The listing builds one solid part. Answer for the finished solid, in the listing's coordinates (mm). A direction names the side the tool comes from. Give positions to 0.01 mm unless a question says otherwise; leave off trailing zeros. Write each loop counter-clockwise with the first axis right and the second up, starting at its lowest first coordinate (ties: lowest second). Pieces come first, ordered by that corner, then holes. Notation, with made-up numbers: M 75,74.5 L 100,74.5 A36 cw 100,111.5 Z; hole C 63,46 d1. An arc over 180 degrees is marked long. Return JSON: item names as keys, results as strings.
from build123d import *

# Parameters (mm, degrees)
SKETCH1_R           = 6.35
BOSS_EXTRUDE1_DEPTH = 17.5
CUT_EXTRUDE1_DEPTH  = 12.8
CHAMFER1_SIZE       = 2
SKETCH4_R           = 3.5
BOSS_EXTRUDE2_DEPTH = 25
SKETCH8_R           = 1.625
CUT_EXTRUDE4_DEPTH  = 30
SKETCH7_R           = 2.5
CUT_EXTRUDE3_DEPTH  = 3.5
SKETCH9_R           = 4
SKETCH9_R_2         = 1.625
BOSS_EXTRUDE3_DEPTH = 5
SKETCH11_R          = 2.75
CUT_EXTRUDE5_DEPTH  = 3
SKETCH12_R          = 1.625
CUT_EXTRUDE6_DEPTH  = 101.436547133
BOSS_EXTRUDE4_DEPTH = 3.7
SKETCH14_R          = 6.35
CUT_EXTRUDE7_DEPTH  = 3.7
CUT_EXTRUDE8_REACH  = 100.805
SKETCH15_W          = 2
SKETCH15_H          = 32.561115391
SKETCH15_H_2        = 13.634806385
SKETCH16_W          = 2
SKETCH16_H          = 5.291502622
CUT_EXTRUDE9_DEPTH  = 20
CUT_EXTRUDE10_REACH = 102.437
SKETCH17_R          = 1.5
CUT_EXTRUDE11_REACH = 102.437
SKETCH18_W          = 1.2
SKETCH18_H          = 8


with BuildPart() as part:
    # Sketch1 → Boss-Extrude1 (new, symmetric)
    with BuildSketch(Plane(origin=(0, 0, 0), x_dir=(0, 0, -1), z_dir=(1, 0, 0))):
        with BuildLine():
            Line((-75, -17.5), (75, -17.5))
            ThreePointArc((75, -17.5), (91.201851746, -6.614378278), (87.247448714, 12.5))
            Line((87.247448714, 12.5), (-69.247448714, 12.5))
            Line((-69.247448714, 12.5), (-69.247448714, 17.5))
            Line((-69.247448714, 17.5), (-75, 17.5))
            ThreePointArc((-75, 17.5), (-92.5, 0), (-75, -17.5))
        make_face()
        with Locations((-75, 0)):
            Circle(SKETCH1_R, mode=Mode.SUBTRACT)
        with Locations((75, 0)):
            Circle(SKETCH1_R, mode=Mode.SUBTRACT)
    extrude(amount=BOSS_EXTRUDE1_DEPTH, both=True)

    # Sketch3 → Cut-Extrude1 (cut, symmetric)
    with BuildSketch(Plane(origin=(0, 0, 0), x_dir=(0, 0, -1), z_dir=(1, 0, 0))):
        with BuildLine():
            Line((-55, -12.5), (75, -12.5))
            ThreePointArc((75, -12.5), (86.858541226, -3.952847075), (82.5, 10))
            Line((82.5, 10), (82.5, 17.5))
            Line((82.5, 17.5), (-92.5, 17.5))
            Line((-92.5, 17.5), (-92.5, -17.5))
            Line((-92.5, -17.5), (-55, -17.5))
            Line((-55, -17.5), (-55, -12.5))
        make_face()
    extrude(amount=CUT_EXTRUDE1_DEPTH, both=True, mode=Mode.SUBTRACT)

    # Chamfer1
    chamfer1_edges = [part.edges().sort_by_distance(p)[0] for p in [
        (17.5, -6.614378278, -91.201851746),
        (17.5, 17.5, 72.123724357),
        (0, -12.5, 55),
        (17.5, 0, 92.5),
        (-17.5, 17.5, 72.123724357),
        (-17.5, -6.614378278, -91.201851746),
        (-17.5, -17.5, 0),
        (-17.5, 0, 92.5),
        (17.5, -17.5, 0),
    ]]
    chamfer(chamfer1_edges, length=CHAMFER1_SIZE)

    # Sketch4 → Boss-Extrude2 (add)
    with BuildSketch(Plane(origin=(0, -12.5, 0), x_dir=(1, 0, 0), z_dir=(0, 1, 0))):
        with Locations((-9.8, 62.5)):
            Circle(SKETCH4_R)
        with Locations((-9.8, 26.333333333)):
            Circle(SKETCH4_R)
        with Locations((-9.8, -9.833333333)):
            Circle(SKETCH4_R)
        with Locations((-9.8, -46)):
            Circle(SKETCH4_R)
    boss_extrude2 = extrude(amount=BOSS_EXTRUDE2_DEPTH)

    # Sketch8 → Cut-Extrude4 (cut)
    with BuildSketch(Plane(origin=(0, 12.5, 0), x_dir=(1, 0, 0), z_dir=(0, 1, 0))):
        with Locations(Location((-9.8, 62.5, 0), (0, 0, 270))):
            Circle(SKETCH8_R)
        with Locations(Location((-9.8, 26.333333333, 0), (0, 0, 270))):
            Circle(SKETCH8_R)
        with Locations(Location((-9.8, -9.833333333, 0), (0, 0, 270))):
            Circle(SKETCH8_R)
        with Locations(Location((-9.8, -46, 0), (0, 0, 270))):
            Circle(SKETCH8_R)
    cut_extrude4 = extrude(amount=-CUT_EXTRUDE4_DEPTH, mode=Mode.SUBTRACT)

    # Sketch7 → Cut-Extrude3 (cut)
    with BuildSketch(Plane.XZ.offset(17.5)):
        with Locations(Location((-9.8, 46, 0), (0, 0, 270))):
            Circle(SKETCH7_R)
        with Locations(Location((-9.8, 9.833333333, 0), (0, 0, 270))):
            Circle(SKETCH7_R)
        with Locations(Location((-9.8, -26.333333333, 0), (0, 0, 270))):
            Circle(SKETCH7_R)
        with Locations(Location((-9.8, -62.5, 0), (0, 0, 270))):
            Circle(SKETCH7_R)
    cut_extrude3 = extrude(amount=-CUT_EXTRUDE3_DEPTH, mode=Mode.SUBTRACT)

    # Sketch9 → Boss-Extrude3 (add, symmetric)
    with BuildSketch(Plane(origin=(0, -12.5, 0), x_dir=(1, 0, 0), z_dir=(0, 1, 0))):
        with Locations((-9.8, 8.25)):
            Circle(SKETCH9_R)
        with Locations(Location((-9.8, 8.25, 0), (0, 0, 270))):
            Circle(SKETCH9_R_2, mode=Mode.SUBTRACT)
    boss_extrude3 = extrude(amount=BOSS_EXTRUDE3_DEPTH, both=True)

    # Sketch11 → Cut-Extrude5 (cut)
    with BuildSketch(Plane.XZ.offset(17.5)):
        with Locations(Location((-9.8, -8.25, 0), (0, 0, 270))):
            Circle(SKETCH11_R)
    cut_extrude5 = extrude(amount=-CUT_EXTRUDE5_DEPTH, mode=Mode.SUBTRACT)

    # Mirror1: Boss-Extrude2, Cut-Extrude4, Cut-Extrude3, Boss-Extrude3, Cut-Extrude5 across plane
    add(boss_extrude2.mirror(Plane(origin=(0, 0, 0), x_dir=(0, 0, 1), z_dir=(1, 0, 0))))
    add(cut_extrude4.mirror(Plane(origin=(0, 0, 0), x_dir=(0, 0, 1), z_dir=(1, 0, 0))), mode=Mode.SUBTRACT)
    add(cut_extrude3.mirror(Plane(origin=(0, 0, 0), x_dir=(0, 0, 1), z_dir=(1, 0, 0))), mode=Mode.SUBTRACT)
    add(boss_extrude3.mirror(Plane(origin=(0, 0, 0), x_dir=(0, 0, 1), z_dir=(1, 0, 0))))
    add(cut_extrude5.mirror(Plane(origin=(0, 0, 0), x_dir=(0, 0, 1), z_dir=(1, 0, 0))), mode=Mode.SUBTRACT)

    # Sketch12 → Cut-Extrude6 (cut, symmetric)
    with BuildSketch(Plane.XZ.offset(17.5)):
        with Locations(Location((9.8, -8.25, 0), (0, 0, 90))):
            Circle(SKETCH12_R)
    cut_extrude6 = extrude(amount=CUT_EXTRUDE6_DEPTH, both=True, mode=Mode.SUBTRACT)

    # Sketch13 → Boss-Extrude4 (add)
    with BuildSketch(Plane(origin=(-12.8, 0, 0), x_dir=(0, 0, -1), z_dir=(1, 0, 0))):
        with BuildLine():
            Line((66.5, 0), (66.5, -12.5))
            Line((66.5, -12.5), (83.5, -12.5))
            Line((83.5, -12.5), (83.5, 0))
            ThreePointArc((83.5, 0), (75, 8.5), (66.5, 0))
        make_face()
    boss_extrude4 = extrude(amount=BOSS_EXTRUDE4_DEPTH)

    # Sketch14 → Cut-Extrude7 (cut)
    with BuildSketch(Plane.ZY.offset(12.8)):
        with Locations(Location((-75, 0, 0), (0, 0, 180))):
            Circle(SKETCH14_R)
    cut_extrude7 = extrude(amount=-CUT_EXTRUDE7_DEPTH, mode=Mode.SUBTRACT)

    # Cut-Extrude8: up to this face of the body (flat: up to its plane)
    cut_extrude8_end = Plane(part.part.faces().sort_by_distance((0.120666671, -12.5, -10.718703908))[0])
    # Sketch15 → Cut-Extrude8 (cut, up to the picked face)
    with BuildSketch(Plane(origin=(0, 12.5, 0), x_dir=(1, 0, 0), z_dir=(0, 1, 0)), mode=Mode.PRIVATE) as cut_extrude8_sk1:
        with Locations((-13.8, 44.416666667)):
            Rectangle(SKETCH15_W, SKETCH15_H)
    cut_extrude8_tool1 = split(extrude(cut_extrude8_sk1.sketch, amount=-CUT_EXTRUDE8_REACH, mode=Mode.PRIVATE), bisect_by=cut_extrude8_end, keep=Keep.BOTH, mode=Mode.PRIVATE)
    # Sketch15 → Cut-Extrude8 (cut, up to the picked face)
    with BuildSketch(Plane(origin=(0, 12.5, 0), x_dir=(1, 0, 0), z_dir=(0, 1, 0)), mode=Mode.PRIVATE) as cut_extrude8_sk2:
        with Locations((-13.8, 17.713154504)):
            Rectangle(SKETCH15_W, SKETCH15_H_2)
    cut_extrude8_tool2 = split(extrude(cut_extrude8_sk2.sketch, amount=-CUT_EXTRUDE8_REACH, mode=Mode.PRIVATE), bisect_by=cut_extrude8_end, keep=Keep.BOTH, mode=Mode.PRIVATE)
    # Sketch15 → Cut-Extrude8 (cut, up to the picked face)
    with BuildSketch(Plane(origin=(0, 12.5, 0), x_dir=(1, 0, 0), z_dir=(0, 1, 0)), mode=Mode.PRIVATE) as cut_extrude8_sk3:
        with Locations((-13.8, -1.213154504)):
            Rectangle(SKETCH15_W, SKETCH15_H_2)
    cut_extrude8_tool3 = split(extrude(cut_extrude8_sk3.sketch, amount=-CUT_EXTRUDE8_REACH, mode=Mode.PRIVATE), bisect_by=cut_extrude8_end, keep=Keep.BOTH, mode=Mode.PRIVATE)
    # Sketch15 → Cut-Extrude8 (cut, up to the picked face)
    with BuildSketch(Plane(origin=(0, 12.5, 0), x_dir=(1, 0, 0), z_dir=(0, 1, 0)), mode=Mode.PRIVATE) as cut_extrude8_sk4:
        with Locations((-13.8, -27.916666666)):
            Rectangle(SKETCH15_W, SKETCH15_H)
    cut_extrude8_tool4 = split(extrude(cut_extrude8_sk4.sketch, amount=-CUT_EXTRUDE8_REACH, mode=Mode.PRIVATE), bisect_by=cut_extrude8_end, keep=Keep.BOTH, mode=Mode.PRIVATE)
    cut_extrude8_1 = cut_extrude8_tool1.solids().sort_by(Axis((-13.8, 12.5, -44.416667), (0, -1, 0)))[0]
    add(cut_extrude8_1, mode=Mode.SUBTRACT)
    cut_extrude8_2 = cut_extrude8_tool2.solids().sort_by(Axis((-13.8, 12.5, -17.713155), (0, -1, 0)))[0]
    add(cut_extrude8_2, mode=Mode.SUBTRACT)
    cut_extrude8_3 = cut_extrude8_tool3.solids().sort_by(Axis((-13.8, 12.5, 1.213155), (0, -1, 0)))[0]
    add(cut_extrude8_3, mode=Mode.SUBTRACT)
    cut_extrude8_4 = cut_extrude8_tool4.solids().sort_by(Axis((-13.8, 12.5, 27.916667), (0, -1, 0)))[0]
    add(cut_extrude8_4, mode=Mode.SUBTRACT)
    cut_extrude8 = cut_extrude8_1 + cut_extrude8_2 + cut_extrude8_3 + cut_extrude8_4  # Cut-Extrude8 as one shape, for the pattern or mirror that repeats it

    # Sketch16 → Cut-Extrude9 (cut)
    with BuildSketch(Plane(origin=(0, 12.5, 0), x_dir=(1, 0, 0), z_dir=(0, 1, 0))):
        with Locations((-13.8, 8.25)):
            Rectangle(SKETCH16_W, SKETCH16_H)
    cut_extrude9 = extrude(amount=-CUT_EXTRUDE9_DEPTH, mode=Mode.SUBTRACT)

    # Mirror2: Cut-Extrude6, Boss-Extrude4, Cut-Extrude7, Cut-Extrude8, Cut-Extrude9 across plane
    add(cut_extrude6.mirror(Plane(origin=(0, 0, 0), x_dir=(0, 0, 1), z_dir=(1, 0, 0))), mode=Mode.SUBTRACT)
    add(boss_extrude4.mirror(Plane(origin=(0, 0, 0), x_dir=(0, 0, 1), z_dir=(1, 0, 0))))
    add(cut_extrude7.mirror(Plane(origin=(0, 0, 0), x_dir=(0, 0, 1), z_dir=(1, 0, 0))), mode=Mode.SUBTRACT)
    add(cut_extrude8.mirror(Plane(origin=(0, 0, 0), x_dir=(0, 0, 1), z_dir=(1, 0, 0))), mode=Mode.SUBTRACT)
    add(cut_extrude9.mirror(Plane(origin=(0, 0, 0), x_dir=(0, 0, 1), z_dir=(1, 0, 0))), mode=Mode.SUBTRACT)

    # Cut-Extrude10: up to this face of the body (flat: up to its plane)
    cut_extrude10_end = Plane(part.part.faces().sort_by_distance((-17.5, -1.343633732, 0.577395586))[0])
    # Sketch17 → Cut-Extrude10 (cut, up to the picked face)
    with BuildSketch(Plane(origin=(17.5, 0, 0), x_dir=(0, 0, -1), z_dir=(1, 0, 0)), mode=Mode.PRIVATE) as cut_extrude10_sk1:
        with Locations((39, 8)):
            Circle(SKETCH17_R)
    cut_extrude10_tool1 = split(extrude(cut_extrude10_sk1.sketch, amount=-CUT_EXTRUDE10_REACH, mode=Mode.PRIVATE), bisect_by=cut_extrude10_end, keep=Keep.BOTH, mode=Mode.PRIVATE)
    add(cut_extrude10_tool1.solids().sort_by(Axis((17.5, 8, -39), (-1, 0, 0)))[0], mode=Mode.SUBTRACT)

    # Cut-Extrude11: up to this face of the body (flat: up to its plane)
    cut_extrude11_end = Plane(part.part.faces().sort_by_distance((17.5, -1.35770743, 0.637008401))[0])
    # Sketch18 → Cut-Extrude11 (cut, up to the picked face)
    with BuildSketch(Plane.ZY.offset(17.5), mode=Mode.PRIVATE) as cut_extrude11_sk1:
        with Locations((-75, 4)):
            Rectangle(SKETCH18_W, SKETCH18_H)
    cut_extrude11_tool1 = split(extrude(cut_extrude11_sk1.sketch, amount=-CUT_EXTRUDE11_REACH, mode=Mode.PRIVATE), bisect_by=cut_extrude11_end, keep=Keep.BOTH, mode=Mode.PRIVATE)
    cut_extrude11 = cut_extrude11_tool1.solids().sort_by(Axis((-17.5, 4, -75), (1, 0, 0)))[0]
    add(cut_extrude11, mode=Mode.SUBTRACT)

    # Mirror3: Cut-Extrude11 across plane
    add(cut_extrude11.mirror(Plane.XY), mode=Mode.SUBTRACT)


solid = part.part
Item 1: Determine the mould class of faces 4 (the cylindrical face through (-16.1, 7.1, -37.8)), 5 (the flat face through (9.1, -7, -75)) for opening direction X: +X half, -X half, draft (parallel to the pull), parting line (faces both ways), or undercut.
Geometry results:
{"face 4": "draft", "face 5": "undercut"}
Item 2: A cutting plane is placed at B-B, the plane x = 1.5. Write down the section's boundary in (y, z), plus the area to 3 significant figures.
Geometry results:
{"outline": "M -17.5,-75 A17.5 ccw 12.5,-87.25 L 12.5,-82.5 L 10,-82.5 A12.5 cw -12.5,-75 L -12.5,53 L -14.5,55 L -17.5,55 Z", "area": "835 mm2"}
Item 3: A cutting plane is placed at A-A, the plane z = -62.5. Write down the section's boundary in (x, y) (3 decimals).
Geometry results:
{"outline": "M -17.5,-15.5 L -15.5,-17.5 L -12.3,-17.5 L -12.3,-14 L -11.425,-14 L -11.425,12.5 L -17.5,12.5 Z; M -8.175,-14 L -7.3,-14 L -7.3,-17.5 L 7.3,-17.5 L 7.3,-14 L 8.175,-14 L 8.175,12.5 L 6.3,12.5 L 6.3,-12.5 L -6.3,-12.5 L -6.3,12.5 L -8.175,12.5 Z; M 11.425,-14 L 12.3,-14 L 12.3,-17.5 L 15.5,-17.5 L 17.5,-15.5 L 17.5,12.5 L 11.425,12.5 Z"}
Item 4: Given pin 1 Ø11.5 at (y, z) = (0, -75) entering from -X; pin 2 Ø1 at (x, y) = (14.5, 2.5) entering from -Z; pin 3 Ø12 at (x, y) = (7, 3.5) entering from +Z; pin 4 Ø1 at (x, y) = (8.5, -1) entering from -Z, each flat-ended and moving along its own axis, determine where each tip first touches the part or whether it passes through.
Geometry results:
{"pin 1": "passes through", "pin 2": "stops at z = -92.39", "pin 3": "stops at z = 92.39", "pin 4": "stops at z = -92.49"}
Item 5: A cutting plane is placed at C-C, the plane z = -8.25. Count the separate pieces of the cut face and the enclosed holes in it, plus the area to 4 significant figures.
Geometry results:
{"separate pieces": "3", "enclosed holes": "0", "area": "317.5 mm2"}
Item 6: Find the intervals of material crossed by line 1 (X direction, y = -15.45, z = -62.5); line 2 (X direction, y = -4, z = 12); line 3 (X direction, y = 4, z = 46) (3 decimals), in increasing order.
Geometry results:
{"line 1": "x = -17.5 to -12.3, -7.3 to 7.3, 12.3 to 17.5", "line 2": "x = -17.5 to -14.8, -12.55 to -7.05, 7.05 to 12.55, 14.8 to 17.5", "line 3": "x = -17.5 to -11.425, -8.175 to -6.3, 6.3 to 8.175, 11.425 to 17.5"}
Item 7: Which of the six approach directions +Z, -Z, +X, -X, +Y, -Y give full straight-line access (tool end or side, diameter ignored) to faces 1 (the cylindrical face through (10.76, -15.77, 43.69)), 2 (the flat face through (11.4, -7.5, -7.4)), 3 (the cylindrical face through (0.179, -4.16, -86.788))?
Geometry results:
{"face 1": "-Y", "face 2": "+Y", "face 3": "none"}
